Geometry check sheet. Reference: drawing and pictorial views, mm from the part's lowest x, y, z. A direction names the side the tool comes from. Coordinates: 2 decimals unless noted, no trailing zeros. Write each loop counter-clockwise with the first axis right and the second up, starting at its lowest first coordinate (ties: lowest second). Pieces come first, ordered by that corner, then holes. Notation, with made-up numbers: (38, -14) -> (59, -14) arc R25 cw to (59, 7) -> close; hole circle Ø11 at (-5.5, -28). An arc over 180 degrees is marked (long way). Use a Markdown table: item, result.
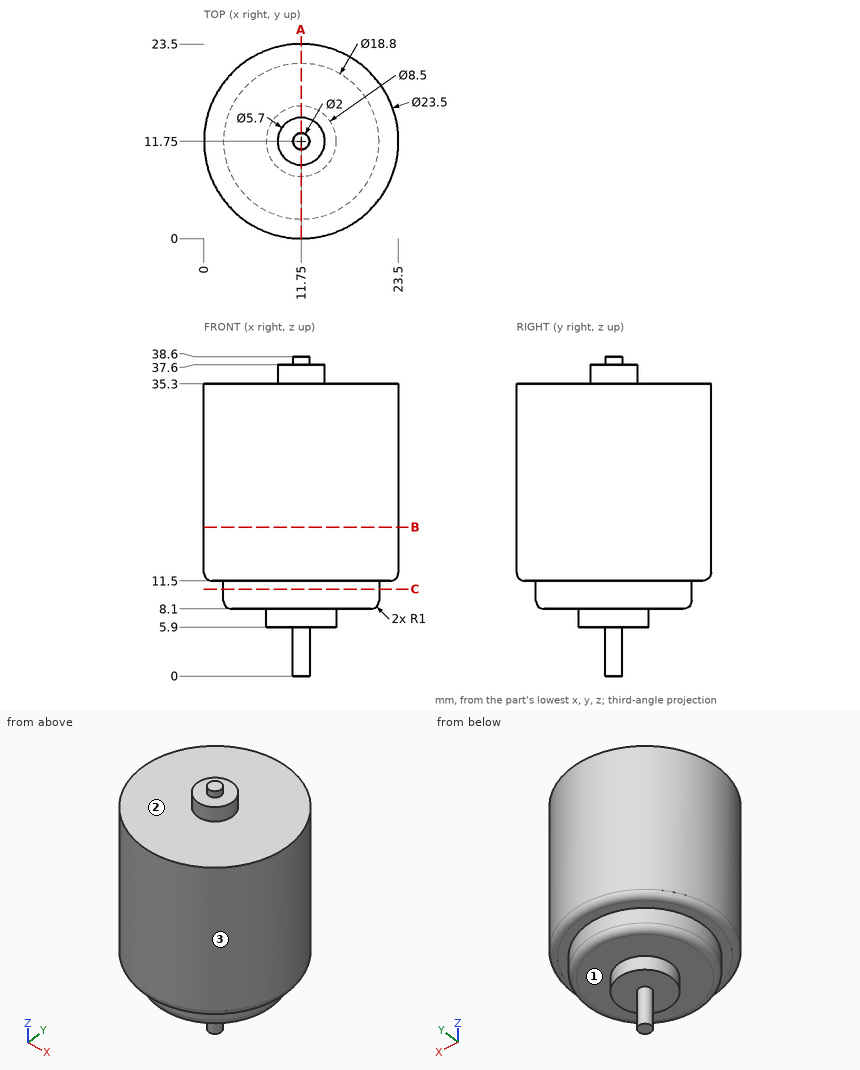
Item 1: Section check A-A on x = 11.75. Record the boundary of the cut face in (y, z), then the cut area to 3 significant figures.
Answer block:
| item | result |
|---|---|
| outline | (0, 12.5) arc R1 ccw to (1, 11.5) -> (2.35, 11.5) -> (2.35, 9.1) arc R1 ccw to (3.35, 8.1) -> (7.5, 8.1) -> (7.5, 5.9) -> (10.75, 5.9) -> (10.75, 0) -> (12.75, 0) -> (12.75, 5.9) -> (16, 5.9) -> (16, 8.1) -> (20.15, 8.1) arc R1 ccw to (21.15, 9.1) -> (21.15, 11.5) -> (22.5, 11.5) arc R1 ccw to (23.5, 12.5) -> (23.5, 35.3) -> (14.6, 35.3) -> (14.6, 37.6) -> (12.75, 37.6) -> (12.75, 38.6) -> (10.75, 38.6) -> (10.75, 37.6) -> (8.9, 37.6) -> (8.9, 35.3) -> (0, 35.3) -> close |
| area | 668 mm^2 |
Item 2: Depth check by flat-ended pin: P1, Ø8, axis at x = 20.5, y = 19.5, coming from the -Z side; P2, Ø6.5, axis at x = 9.5, y = 8, coming from the -Z side; P3, Ø10, axis at x = 3, y = 8, coming from the +Z side; P4, Ø1.7, axis at x = 10.5, y = 12.5, coming from the +Z side. Enter the tip coordinate at first touch or a pass-through.
Answer block:
| item | result |
|---|---|
| P1 | stops at z = 8.1 |
| P2 | stops at z = 5.9 |
| P3 | stops at z = 35.3 |
| P4 | stops at z = 38.6 |
Item 3: Thickness scan on L1, parallel to Z at x = 7.75, y = 6.75; L2, parallel to Z at x = 2, y = 8.75; L3, parallel to X at y = 16, z = 28. Record the ranges inside material, lowest first. Write a range as [from, to].
Answer block:
| item | result |
|---|---|
| L1 | z = [8.1, 35.3] |
| L2 | z = [11.5, 35.3] |
| L3 | x = [0.8, 22.7] |
Item 4: Tool access check on the marked faces 1, 2 and 3. Record the directions out of +Z, -Z, +X, -X, +Y, -Y that give a thin tool (end or side, any length) a straight path to the whole face; none if there is none.
Answer block:
| item | result |
|---|---|
| face 1 | -Z |
| face 2 | +Z |
| face 3 | +Z, -Z |
Item 5: Section check B-B on z = 18. Record the boundary of the cut face in (x, y), then the cut area to 3 significant figures.
Answer block:
| item | result |
|---|---|
| outline | circle Ø23.5 at (11.75, 11.75) |
| area | 434 mm^2 |
Item 6: Section check C-C on z = 10.5. Record the boundary of the cut face in (x, y), then the cut area to 3 significant figures.
Answer block:
| item | result |
|---|---|
| outline | circle Ø18.8 at (11.75, 11.75) |
| area | 278 mm^2 |
